```python
from build123d import *

# Parameters (mm, degrees)
SKETCH1_R                    = 48
BOSS_EXTRUDE1_DEPTH          = 2
SKETCH3_R                    = 2
CUT_EXTRUDE1_DEPTH           = 68.911707385
SKETCH2_R                    = 0.825
CUT_EXTRUDE_NANO_RECTO_DEPTH = 68.911707385
SKETCH4_R                    = 0.825
CUT_EXTRUDE_VERSO_DEPTH      = 68.911707385


with BuildPart() as part:
    # Sketch1 → Boss-Extrude1 (new body)
    with BuildSketch(Plane.XY):
        Circle(SKETCH1_R)
    extrude(amount=BOSS_EXTRUDE1_DEPTH)

    # Sketch3 → Cut-Extrude1 (cut, through all)
    with BuildSketch(Plane(origin=(0, 0, 0), x_dir=(-1, 0, 0), z_dir=(0, 0, -1))):
        with Locations((30.405591591, 30.405591591)):
            Circle(SKETCH3_R)
        with Locations((11.129218939, -41.53481053)):
            Circle(SKETCH3_R)
        with Locations((-41.53481053, 11.129218939)):
            Circle(SKETCH3_R)
    extrude(amount=-CUT_EXTRUDE1_DEPTH, mode=Mode.SUBTRACT)

    # Sketch2 → Cut-Extrude-Nano+Recto (cut, through all)
    with BuildSketch(Plane.XY.offset(2)):
        with Locations((20.32, 38.74)):
            Circle(SKETCH2_R)
        with Locations(Location((20.32, 23.5, 0), (0, 0, 180))):
            Circle(SKETCH2_R)
        with Locations((-20.32, 23.5)):
            Circle(SKETCH2_R)
        with Locations(Location((-20.32, 38.74, 0), (0, 0, 180))):
            Circle(SKETCH2_R)
        with Locations((34.74, 18.98)):
            Circle(SKETCH2_R)
        with Locations(Location((6.26, 18.98, 0), (0, 0, 180))):
            Circle(SKETCH2_R)
        with Locations((-39.24, 18.98)):
            Circle(SKETCH2_R)
        with Locations(Location((1.24, 18.98, 0), (0, 0, 180))):
            Circle(SKETCH2_R)
        with Locations((1.24, -21.5)):
            Circle(SKETCH2_R)
        with Locations(Location((-39.24, -21.5, 0), (0, 0, 180))):
            Circle(SKETCH2_R)
        with BuildLine():
            Line((17.78, 23), (-17.78, 23))
            ThreePointArc((-17.78, 23), (-18.28, 23.5), (-17.78, 24))
            Line((-17.78, 24), (17.78, 24))
            ThreePointArc((17.78, 24), (18.28, 23.5), (17.78, 23))
        make_face()
        with BuildLine():
            Line((17.78, 39.24), (-17.78, 39.24))
            ThreePointArc((-17.78, 39.24), (-18.28, 38.74), (-17.78, 38.24))
            Line((-17.78, 38.24), (17.78, 38.24))
            ThreePointArc((17.78, 38.24), (18.28, 38.74), (17.78, 39.24))
        make_face()
    extrude(amount=-CUT_EXTRUDE_NANO_RECTO_DEPTH, mode=Mode.SUBTRACT)

    # Sketch4 → Cut-Extrude-Verso (cut, through all)
    with BuildSketch(Plane(origin=(0, 0, 0), x_dir=(-1, 0, 0), z_dir=(0, 0, -1))):
        with Locations((-8.26, -36.34)):
            Circle(SKETCH4_R)
        with Locations((2.18, -36.34)):
            Circle(SKETCH4_R)
        with Locations(Location((-26.13, -36.34, 0), (0, 0, 180))):
            Circle(SKETCH4_R)
        with Locations((20.48, -24.54)):
            Circle(SKETCH4_R)
        with BuildLine():
            Line((11.68, -36.34), (11.68, -25.34))
            ThreePointArc((11.68, -25.34), (12.18, -24.84), (12.68, -25.34))
            Line((12.68, -25.34), (12.68, -36.34))
            ThreePointArc((12.68, -36.34), (12.18, -36.84), (11.68, -36.34))
        make_face()
    extrude(amount=-CUT_EXTRUDE_VERSO_DEPTH, mode=Mode.SUBTRACT)


solid = part.part
```
Check sheet for the modelled part. Datum: model origin and axes. Units: mm. Give positions to 0.01 mm unless a question says otherwise; leave off trailing zeros. Order: outer loops, then holes, each group sorted by start corner. A loop starts at its lowest first (then second) coordinate and runs counter-clockwise, first axis right, second up. Notation, with made-up numbers: M 60,77.5 L 104,77.5 A16 cw 104,84.5 Z; hole C 87,31.25 d2. An arc over 180 degrees is marked long. Answer in a Markdown table with one row per item.
1) Cross-section at A-A, the plane y = -30. Enter the section's corners in (x, z), plus the area to 3 significant figures.
Filled sheet:
| item | result |
|---|---|
| outline | M -37.47,0 L -12.68,0 L -12.68,2 L -37.47,2 Z; M -11.68,0 L 37.47,0 L 37.47,2 L -11.68,2 Z |
| area | 148 mm2 |
2) Cross-section at B-B, the plane x = -15. Enter the section's corners in (y, z), plus the area to 3 significant figures.
Filled sheet:
| item | result |
|---|---|
| outline | M -45.6,0 L 23,0 L 23,2 L -45.6,2 Z; M 24,0 L 38.24,0 L 38.24,2 L 24,2 Z; M 39.24,0 L 45.6,0 L 45.6,2 L 39.24,2 Z |
| area | 178 mm2 |
3) Cross-section at C-C, the plane z = 0.75. Count the separate pieces of the cut face and the enclosed holes in it, plus the area to 3 significant figures.
Filled sheet:
| item | result |
|---|---|
| separate pieces | 1 |
| enclosed holes | 20 |
| area | 7,090 mm2 |
4) Thickness scan on L1, parallel to Y at x = 0, z = 1.5; L2, parallel to X at y = -36.34, z = 1.15 (3 decimals); L3, parallel to Y at x = 6, z = 0.55. Record the ranges inside material, lowest first. Write a range as [from, to].
Filled sheet:
| item | result |
|---|---|
| L1 | y = [-48, 23], [24, 38.24], [39.24, 48] |
| L2 | x = [-31.359, -12.68], [-11.68, -3.005], [-1.355, 7.435], [9.085, 25.305], [26.955, 31.359] |
| L3 | y = [-47.62, 18.2], [19.76, 23], [24, 38.24], [39.24, 47.62] |
5) Release check for a two-part mould opening along Y. For faces 1 (the cylindrical face through (-10.7, -43.49, 0.99)), 2 (the flat face through (-1, 1, 0)), 3 (the cylindrical face through (-47.954, 2.11, 0.986)), 4 (the cylindrical face through (-30.15, 32.39, 0.99)) record: +Y half, -Y half, draft (parallel to the pull), parting line (faces both ways), or undercut.
Filled sheet:
| item | result |
|---|---|
| face 1 | undercut |
| face 2 | draft |
| face 3 | parting line |
| face 4 | undercut |
6) Cross-section at D-D, the plane x = -37. Enter the section's corners in (y, z).
Filled sheet:
| item | result |
|---|---|
| outline | M -30.58,0 L 30.58,0 L 30.58,2 L -30.58,2 Z |
7) Gauge pin test, flat ends, axial feed: P1, Ø1, axis at y = 27, z = 0.5, coming from the +X side; P2, Ø0.6, axis at x = 1, z = 1, coming from the +Y side; P3, Ø0.6, axis at x = 6.5, z = 1, coming from the +Y side. Record the tip position at first contact, or that the pin passes through.
Filled sheet:
| item | result |
|---|---|
| P1 | stops at x = 40.02 |
| P2 | stops at y = 47.99 |
| P3 | stops at y = 47.6 |
